Study the drawing (mm; zero at the part's minimum x, y, z) and answer. Coordinates: 2 decimals unless noted, no trailing zeros. Order: outer loops, then holes, each group sorted by start corner. A loop starts at its lowest first (then second) coordinate and runs counter-clockwise, first axis right, second up. Notation, with made-up numbers: (-19, 68.5) -> (2, 68.5) arc R25 cw to (2, 95.5) -> close; hole circle Ø3 at (-1, 78). An arc over 180 degrees is marked (long way). Write each question's results on one line, items separated by ' | '. Start each with the question number.
(1) Given pin 1 (10 mm diameter, centred on y = 17, z = 31.5, fed in from +X); pin 2 (12 mm diameter, centred on x = 17.5, z = 28, fed in from -Y); pin 3 (6.5 mm diameter, centred on x = 9, y = 12.5, fed in from +Z), each flat-ended and moving along its own axis, determine where each tip first touches the part or whether it passes through.
(2) The part is cut by section A-A, the plane x = 9. Give the vertices of the cut face in (y, z).
(3) The part is cut by section C-C, the plane z = 4.5. Give the vertices of the cut face in (x, y).
(4) Straight lines are drawn through the part: L1, parallel to Y at x = 31, z = 6; L2, parallel to Y at x = 3.5, z = 26; L3, parallel to X at y = 12, z = 9. For each, find the intervals that lie inside material, in ascending order.
(5) The part is cut by section D-D, the plane x = 4. Give the vertices of the cut face in (y, z).
(6) Determine the mould class of the marked faces 1, 2 and 3 for opening direction Z: +Z half, -Z half, draft (parallel to the pull), parting line (faces both ways), or undercut.
(7) The part is cut by section B-B, the plane y = 12.5. Give the vertices of the cut face in (x, z), then the cut area to 3 significant figures.
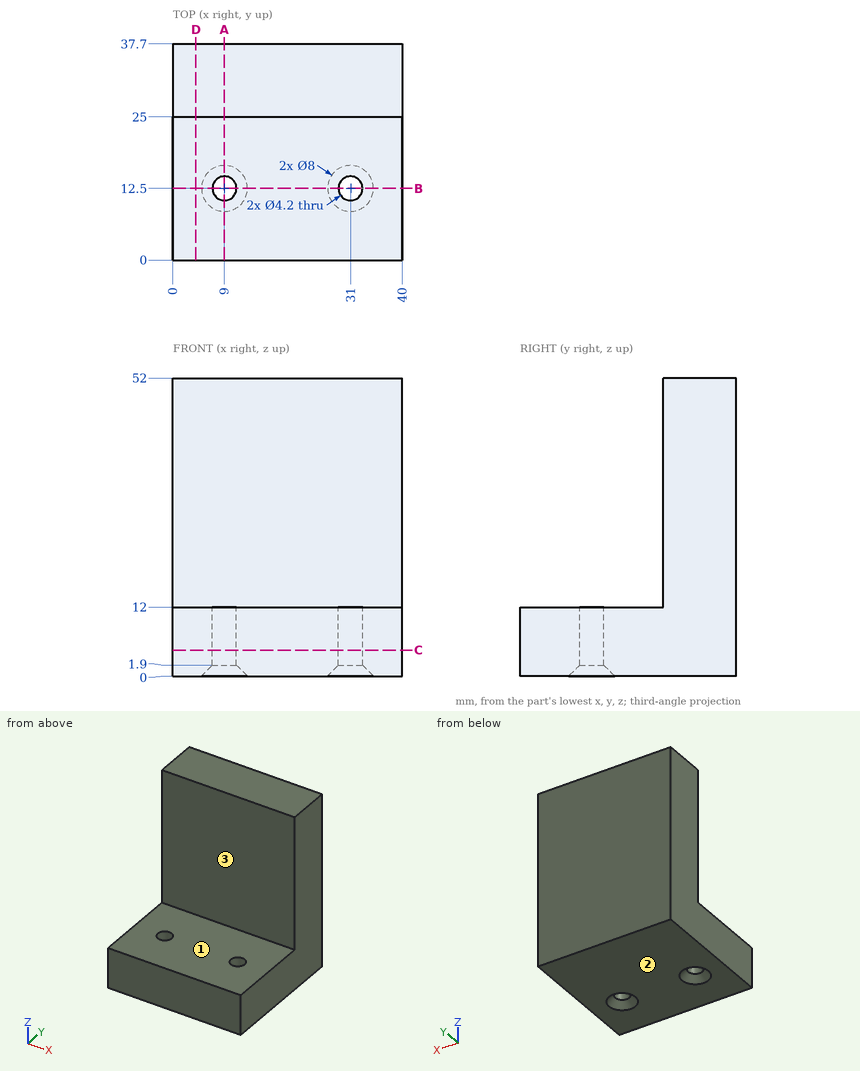
Established:
1) pin 1: passes through | pin 2: stops at y = 25 | pin 3: stops at z = 12
2) outline: (0, 0) -> (8.5, 0) -> (10.4, 1.9) -> (10.4, 12) -> (0, 12) -> close; (14.6, 1.9) -> (16.5, 0) -> (37.7, 0) -> (37.7, 52) -> (25, 52) -> (25, 12) -> (14.6, 12) -> close
3) outline: (0, 0) -> (40, 0) -> (40, 37.7) -> (0, 37.7) -> close; hole circle Ø4.2 at (9, 12.5); hole circle Ø4.2 at (31, 12.5)
4) L1: y = 0 to 10.4, 14.6 to 37.7 | L2: y = 25 to 37.7 | L3: x = 0 to 6.96, 11.04 to 28.96, 33.04 to 40
5) outline: (0, 0) -> (37.7, 0) -> (37.7, 52) -> (25, 52) -> (25, 12) -> (0, 12) -> close
6) face 1: +Z half | face 2: -Z half | face 3: draft
7) outline: (0, 0) -> (5, 0) -> (6.9, 1.9) -> (6.9, 12) -> (0, 12) -> close; (11.1, 1.9) -> (13, 0) -> (27, 0) -> (28.9, 1.9) -> (28.9, 12) -> (11.1, 12) -> close; (33.1, 1.9) -> (35, 0) -> (40, 0) -> (40, 12) -> (33.1, 12) -> close | area: 372 mm^2
